```python
from build123d import *

# Parameters (mm, degrees)
CHAMFER1_SIZE      = 0.22
CHAMFER1_SIZE2     = 0.381051178
CUT_EXTRUDE1_DEPTH = 0.8
CUT_EXTRUDE1_TAPER = 6


with BuildPart() as part:
    # Sketch1 → Revolve1 (revolve)
    with BuildSketch(Plane.XY, mode=Mode.PRIVATE) as revolve1_sk:
        with BuildLine():
            Line((0, 2), (-0.897999199, 2))
            ThreePointArc((-0.897999199, 2), (-1.419403703, 1.059811908), (-1.6, 0))
            Line((-1.6, 0), (4.5, 0))
            Line((4.5, 0), (4.5, 1.1))
            Line((4.5, 1.1), (0, 1.1))
            Line((0, 1.1), (0, 2))
        make_face()
    revolve(revolve1_sk.sketch.rotate(Axis((0, 0, 0), (1, 0, 0)), 90), axis=Axis((0, 0, 0), (1, 0, 0)))

    # Chamfer1
    chamfer1_edges = [part.edges().sort_by_distance(p)[0] for p in [
        (4.5, 0, -1.1),
    ]]
    chamfer1_side = [part.faces().sort_by_distance(p)[0] for p in [
        (4.5, 0, 0),
    ]]
    chamfer(chamfer1_edges, length=CHAMFER1_SIZE, length2=CHAMFER1_SIZE2, reference=chamfer1_side[0])

    # Sketch3 → Cut-Extrude1 (cut)
    with BuildSketch(Plane(origin=(-1.6, 0, 0), x_dir=(0, 0, -1), z_dir=(1, 0, 0))):
        Polygon((-0.2375, 0.95), (-0.1425, 0.57), (-0.29897586, 0.29897586), (-0.57, 0.1425), (-0.95, 0.2375), (-0.95, -0.2375), (-0.57, -0.1425), (-0.29897586, -0.29897586), (-0.1425, -0.57), (-0.2375, -0.95), (0.2375, -0.95), (0.1425, -0.57), (0.29897586, -0.29897586), (0.57, -0.1425), (0.95, -0.2375), (0.95, 0.2375), (0.57, 0.1425), (0.29897586, 0.29897586), (0.1425, 0.57), (0.2375, 0.95), align=None)
    extrude(amount=CUT_EXTRUDE1_DEPTH, taper=CUT_EXTRUDE1_TAPER, mode=Mode.SUBTRACT)


solid = part.part
```
Can you work these out from the model? Positions are in its coordinate system, mm. Give positions to 0.01 mm unless a question says otherwise; leave off trailing zeros. Loops run counter-clockwise (first coordinate to the right, second up) from the corner with the lowest first, then second, coordinate; pieces in that order, holes last. Notation, with made-up numbers: M 39,15.5 L 90,15.5 A28 ccw 90,39.5 Z; hole C 8.25,15.25 d7. An arc over 180 degrees is marked long. One line per item, written item: value.
(1) I need wall thicknesses on line 1 (Z direction, x = -0.25, y = -0.4); line 2 (X direction, y = 1.1, z = -1.15); line 3 (X direction, y = 1.65, z = 0.35). Which ranges of each line are inside material? Lowest first, please.
Returned:
line 1: -1.96 to 1.96
line 2: -1.18 to 0
line 3: -1.12 to 0
(2) Will this pin go through, and if not, where does the flat tip stop? pin 1 (1.5 mm diameter, centred on x = 3, z = 1.5, fed in from -Y).
Returned:
pin 1: y = -0.8
(3) Suppose I cut it at C-C on z = 1.75. List the corners of the cut face in (x, y) for me.
Returned:
outline: M -0.9,-0.97 L 0,-0.97 L 0,0.97 L -0.9,0.97 A2.68 ccw Z
(4) Suppose I cut it at A-A on x = 0.25. List the corners of the cut face in (y, z) for me, plus the area to 3 significant figures.
Returned:
outline: C 0,0 d2.2
area: 3.80 mm^2
(5) Suppose I cut it at B-B on z = -1.2. List the corners of the cut face in (x, y) for me, plus the area to 3 significant figures.
Returned:
outline: M -0.9,-1.6 L 0,-1.6 L 0,1.6 L -0.9,1.6 A2.97 ccw Z
area: 3.89 mm^2
(6) We'd pull the mould along Z, two halves only. Please class faces 1 (the face through (-0.8, 0, 0)), 2 (the face through (-0.455, 1.952, -0.434)), 3 (the face through (4.5, 0, 0)): released by +Z, released by -Z, zero draft, split by the parting line, or undercut.
Returned:
face 1: undercut
face 2: split by the parting line
face 3: zero draft
